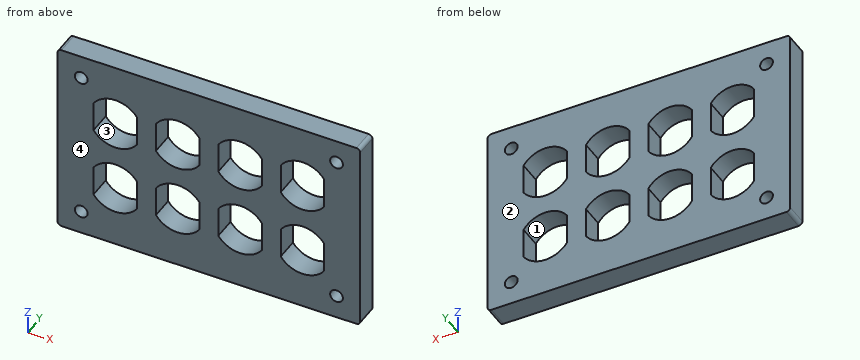
Autodesk Inventor part; units mm, degrees
ref_plane "YZ Plane" through (0, 0, 0) normal (1, 0, 0) x (0, 1, 0)
ref_plane "XZ Plane" through (0, 0, 0) normal (0, 1, 0) x (-1, 0, 0)
ref_plane "XY Plane" through (0, 0, 0) normal (0, 0, 1) x (1, 0, 0)
sketch "Sketch1" plane through (0, 0, 0) normal (0, 1, 0) x (-1, 0, 0)
  line L0 (80, 52) -> (-80, 52)
  line L1 (-80, 52) -> (-80, -52)
  line L2 (-80, -52) -> (80, -52)
  line L3 (80, -52) -> (80, 52)
  line L4 (80, 52) -> (-80, -52) construction
  line L5 (-80, 52) -> (80, -52) construction
  point P0 (0, 0)
  dimension "d0" = 160
  dimension "d1" = 104
extrude "Extrusion1" add sketch "Sketch1" along normal blind 12
sketch "Sketch2" plane through (0, 12, 0) normal (0, 1, 0) x (1, 0, 0)
  line L0 (-38, 27) -> (-38, 11)
  line L1 (-61, 11) -> (-61, 27)
  line L2 (-80, 52) -> (-80, -52)
  line L3 (80, 52) -> (-80, 52)
  arc A0 (-38, 27) -> (-61, 27) centre (-49.5, 19) ccw
  arc A1 (-61, 11) -> (-38, 11) centre (-49.5, 19) ccw
  point P0 (0, 0)
  dimension "d4" = 23
  dimension "d5" = 16
  dimension "d6" = 19
  dimension "d8" = 33
extrude "Extrusion2" cut sketch "Sketch2" against normal up to next
pattern_linear "Rectangular Pattern1" count 4 spacing -33 along (-1, 0, 0) count 2 spacing 38 along (0, 0, 1) of "Extrusion2"
sketch "Sketch4" plane through (0, 12, 0) normal (0, 1, 0) x (1, 0, 0)
  line L0 (-80, 52) -> (-80, -52)
  line L1 (80, 52) -> (-80, 52)
  line L2 (80, -52) -> (80, 52)
  line L3 (-80, -52) -> (80, -52)
  point P0 (0, 0)
  point P1 (-67.5, 39.5)
  point P2 (67.5, 39.5)
  point P3 (67.5, -39.5)
  point P4 (-67.5, -39.5)
  dimension "d24" = 12.5
  dimension "d25" = 12.5
  dimension "d26" = 12.5
  dimension "d27" = 12.5
  dimension "d28" = 12.5
  dimension "d29" = 12.5
  dimension "d30" = 12.5
  dimension "d31" = 12.5
hole "Hole1" at (-67.5, 12, -39.5) at (67.5, 12, -39.5) at (67.5, 12, 39.5) at (-67.5, 12, 39.5) direction (0, -1, 0) diameter 6.756 depth 25.4
fillet "Fillet1" radius 2 4 edges at (-80, 6, 52) (80, 6, 52) (80, 6, -52) (-80, 6, -52)
properties part number "4_OM_VialPlate"
The model under review builds one solid part; all positions refer to its coordinate system, in mm. Face numbers are marked on the shaded views. A direction names the side the tool comes from. Coordinates: 2 decimals unless noted, no trailing zeros. Write each loop counter-clockwise with the first axis right and the second up, starting at its lowest first coordinate (ties: lowest second). Pieces come first, ordered by that corner, then holes. Notation, with made-up numbers: M -18.5,82 L 16.5,82 A21 ccw 16.5,108 Z; hole C 9,42.25 d1. An arc over 180 degrees is marked long. Put each result on its own line as item: value.
1) Add section C-C on z = 13.5. Give the boundary of the cut face in (x, y), then the cut area to 3 significant figures.
Computed:
outline: M -80,0 L -61,0 L -61,12 L -80,12 Z; M -38,0 L -28,0 L -28,12 L -38,12 Z; M -5,0 L 5,0 L 5,12 L -5,12 Z; M 28,0 L 38,0 L 38,12 L 28,12 Z; M 61,0 L 80,0 L 80,12 L 61,12 Z
area: 816 mm2
2) Add section B-B on z = -39.5. Give the boundary of the cut face in (x, y).
Computed:
outline: M -80,0 L -70.88,0 L -70.88,12 L -80,12 Z; M -64.12,0 L 64.12,0 L 64.12,12 L -64.12,12 Z; M 70.88,0 L 80,0 L 80,12 L 70.88,12 Z
3) Wall thickness on probe 1 along Z at (x, y) = (67.5, 4); probe 2 along X at (y, z) = (9.25, 12); probe 3 along X at (y, z) = (7.5, -39.5): over which ranges is each line inside the solid? List them lowest first. Write a range as [from, to].
Computed:
probe 1: z = [-52, -42.88], [-36.12, 36.12], [42.88, 52]
probe 2: x = [-80, -61], [-38, -28], [-5, 5], [28, 38], [61, 80]
probe 3: x = [-80, -70.88], [-64.12, 64.12], [70.88, 80]
4) For the marked faces 3 and 4, list the 3-axis set-ups (+Z, -Z, +X, -X, +Y, -Y) from which the entire face can be reached by the end or side of a thin tool; tool diameter is ignored.
Computed:
face 3: +Y, -Y
face 4: +Z, -Z, +X, -X, -Y
5) Add section A-A on x = -67.5. Give the boundary of the cut face in (y, z), then the cut area to 3 significant figures.
Computed:
outline: M 0,-52 L 12,-52 L 12,-42.88 L 0,-42.88 Z; M 0,-36.12 L 12,-36.12 L 12,36.12 L 0,36.12 Z; M 0,42.88 L 12,42.88 L 12,52 L 0,52 Z
area: 1,090 mm2
6) Add section D-D on y = 3. State how many separate pieces and enclosed holes the cut face has, then the cut area to 3 significant figures.
Computed:
separate pieces: 1
enclosed holes: 12
area: 12,000 mm2
7) Draft analysis for pull direction X (two halves, no side actions). For the marked faces 1 and 2, state which applies: released by +X, released by -X, zero draft, split by the parting line, or undercut.
Computed:
face 1: undercut
face 2: zero draft
